Autodesk Inventor part; units mm, degrees
ref_plane "YZ Plane" through (0, 0, 0) normal (1, 0, 0) x (0, 1, 0)
ref_plane "XZ Plane" through (0, 0, 0) normal (0, 1, 0) x (-1, 0, 0)
ref_plane "XY Plane" through (0, 0, 0) normal (0, 0, 1) x (1, 0, 0)
sketch "Sketch1" plane through (0, 0, 0) normal (1, 0, 0) x (0, 1, 0)
  circle A0 centre (0, 0) radius 4
  dimension "d0" = 8
extrude "Extrusion1" add sketch "Sketch1" along normal blind 25
sketch "Sketch3" plane through (25, 0, 0) normal (1, 0, 0) x (0, 0, -1)
  point P0 (0, 0)
  point P1 (0, 0)
hole "Hole1" at (25, -0.0356, 0.0036) direction (-1, 0, 0) diameter 4.134 depth 10
sketch "Sketch4" plane through (0, 0, 0) normal (-1, 0, 0) x (0, 0, 1)
  point P0 (0, 0)
  point P1 (0, 0)
hole "Hole2" at (0, 0, 0) direction (1, 0, 0) diameter 4.917 depth 10
properties part number "CopleCylinderSensor"
For this review, take the finished solid that the model builds, in its own axes (mm). A direction names the side the tool comes from. Coordinates: 2 decimals unless noted, no trailing zeros. Write each loop counter-clockwise with the first axis right and the second up, starting at its lowest first coordinate (ties: lowest second). Pieces come first, ordered by that corner, then holes. Notation, with made-up numbers: (-30.75, -9) - (3.25, -9) arc R26 ccw to (3.25, 16) - close; hole circle Ø4 at (-35, 46). An arc over 180 degrees is marked (long way). Answer in a Markdown table with one row per item. Add a question column.
Q1. We need section C-C, the plane x = 5.25. State the section outline as (y, z) points, and give its area (3 significant figures).
Q2. Draft analysis for pull direction Z (two halves, no side actions). For faces 4 (the flat face through (0, 2, 2)), 5 (the cylindrical face through (12.325, -0.867, 3.905)), 6 (the cylindrical face through (5.07, -0.738, 2.345)), state which applies: +Z half, -Z half, draft (parallel to the pull), parting line (faces both ways), or undercut.
Q3. We need section A-A, the plane z = 0. State the section outline as (x, y) points, and give its area (3 significant figures).
Q4. For P1, Ø1, axis at x = 3.5, y = 2.5, coming from the -Z side; P2, Ø1, axis at x = 8.5, z = -1, coming from the +Y side, all flat-tipped, find the tip position at first contact; note any pin that passes through.
Q5. Tool access review of faces 1 (the flat face through (10, 0, 0)), 2 (the cylindrical face through (19.93, 1.222, 1.644)), 3 (the flat face through (25, 2, -2)): name each direction out of +Z, -Z, +X, -X, +Y, -Y from which nothing blocks a thin tool from reaching the whole face with its end or side.
Q6. We need section D-D, the plane x = 20.75. State the section outline as (y, z) points.
Q7. We need section B-B, the plane y = -1.75. State the section outline as (x, z) points, and give its area (3 significant figures).
Q8. For probe 1 along Z at (x, y) = (3.5, 0); probe 2 along Z at (x, y) = (17.5, 0); probe 3 along Y at (x, z) = (7.75, 1.5), list the stretches that pass through material, from the lowest coordinate up.
Answer list:
| question | item | result |
|---|---|---|
| 1 | outline | circle Ø8 at (0, 0); hole circle Ø4.92 at (0, 0) |
| 1 | area | 31.3 mm2 |
| 2 | face 4 | draft |
| 2 | face 5 | parting line |
| 2 | face 6 | undercut |
| 3 | outline | (0, -4) - (25, -4) - (25, -2.1) - (15, -2.1) - (15, 2.03) - (25, 2.03) - (25, 4) - (0, 4) - (0, 2.46) - (10, 2.46) - (10, -2.46) - (0, -2.46) - close |
| 3 | area | 109 mm2 |
| 4 | P1 | stops at z = -3.46 |
| 4 | P2 | stops at y = 3.97 |
| 5 | face 1 | -X |
| 5 | face 2 | +X |
| 5 | face 3 | +Z, -Z, +X, +Y, -Y |
| 6 | outline | circle Ø8 at (0, 0); hole circle Ø4.13 at (-0.04, 0) |
| 7 | outline | (0, -3.6) - (25, -3.6) - (25, -1.15) - (15, -1.15) - (15, 1.16) - (25, 1.16) - (25, 3.6) - (0, 3.6) - (0, 1.73) - (10, 1.73) - (10, -1.73) - (0, -1.73) - close |
| 7 | area | 122 mm2 |
| 8 | probe 1 | z = -4 to -2.46, 2.46 to 4 |
| 8 | probe 2 | z = -4 to -2.06, 2.07 to 4 |
| 8 | probe 3 | y = -3.71 to -1.95, 1.95 to 3.71 |
